The model under review builds one solid part; all positions refer to its coordinate system, in mm. Face numbers are marked on the shaded views. A direction names the side the tool comes from. Round coordinates to 2 decimals unless told otherwise and drop trailing zeros. Order: outer loops, then holes, each group sorted by start corner. A loop starts at its lowest first (then second) coordinate and runs counter-clockwise, first axis right, second up. Notation, with made-up numbers: M -6,40 L 43,40 A10 cw 43,56 Z; hole C 61.25,-23.75 d1. An arc over 180 degrees is marked long. Use a Markdown table: item, result. Add a question column.
1. For the marked faces 1, 2, 3, 4 and 5, list the 3-axis set-ups (+Z, -Z, +X, -X, +Y, -Y) from which the entire face can be reached by the end or side of a thin tool; tool diameter is ignored.
2. Consider section A-A on y = -43. State the section outline as (x, z) points.
3. The part is to be moulded in two halves that separate along Y. For the marked faces 6, 7, 8 and 9, say which applies: +Y half, -Y half, draft (parallel to the pull), parting line (faces both ways), or undercut.
4. Consider section C-C on x = 45. State the section outline as (y, z) points, then the cut area to 3 significant figures.
5. Consider section D-D on z = 22.5. State the section outline as (x, y) points.
6. Consider section B-B on z = 5.5. State the section outline as (x, y) points.
7. Insertion check: P1, Ø9, axis at x = -18, y = -40, coming from the +Z side; P2, Ø10, axis at x = 38.5, z = 22.5, coming from the -Y side; P3, Ø16.5, axis at x = 10.5, y = -27, coming from the +Z side; P4, Ø8, axis at x = 1, z = 15, coming from the +Y side. Each pin has a flat end and moves straight along its axis. Give the tip position at first contact, or say it passes through.
8. To check wall thickness, follow probe 1 along Y at (x, z) = (25.5, 0.5); probe 2 along Y at (x, z) = (0, 37.5); probe 3 along Z at (x, y) = (-11.5, -33). State the ranges of each line that lie inside material, in increasing order.
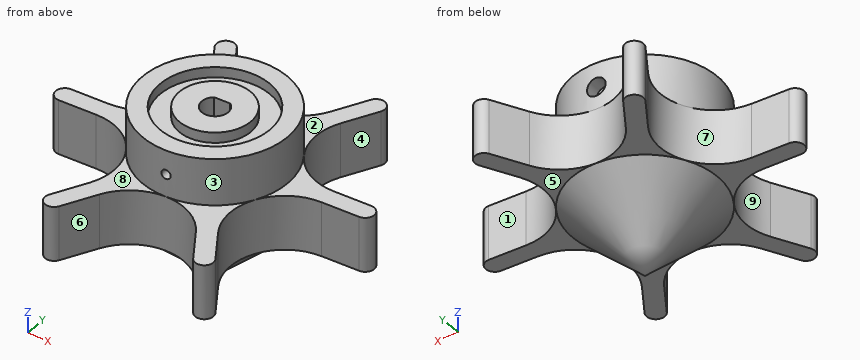
from build123d import *

# Parameters (mm, degrees)
SKETCH1_R               = 3.5
BOSS_EXTRUDE1_DEPTH     = 21
SKETCH4_R               = 28
BOSS_EXTRUDE2_DEPTH     = 18
SKETCH6_R               = 21.2
SKETCH6_R_2             = 13.8
CUT_EXTRUDE1_DEPTH      = 4
CUT_EXTRUDE2_DEPTH      = 20
CUT_EXTRUDE3_DEPTH      = 93.206949894
CUT_EXTRUDE3_DEPTH_BACK = 93.206949894
SKETCH7_R               = 1.75
SKETCH8_R               = 3.5
CUT_EXTRUDE4_DEPTH      = 5.5


with BuildPart() as part:
    # Sketch1 → Boss-Extrude1 (new body)
    with BuildSketch(Plane.XY):
        with BuildLine():
            ThreePointArc((-27.16441994, 47.550254291), (-29.67571676, 44.192804958), (-33.605829095, 45.653385243))
            Line((-33.605829095, 45.653385243), (-25.93972411, 33.765821671))
            ThreePointArc((-25.93972411, 33.765821671), (-24.90753088, 12.791204222), (-42.555985811, 1.409989939))
            Line((-42.555985811, 1.409989939), (-56.683970347, 0.71473006))
            ThreePointArc((-56.683970347, 0.71473006), (-54.098653318, -0.246072778), (-53.011938142, -2.781039515))
            ThreePointArc((-53.011938142, -2.781039515), (-53.976971405, -5.194324339), (-56.339905937, -6.27680909))
            Line((-56.339905937, -6.27680909), (-42.211921401, -5.581549211))
            ThreePointArc((-42.211921401, -5.581549211), (-23.531273241, -15.174952377), (-22.499080012, -36.149569826))
            Line((-22.499080012, -36.149569826), (-28.960959562, -48.732393278))
            ThreePointArc((-28.960959562, -48.732393278), (-25.025035607, -46.929305801), (-22.347518202, -50.331293805))
            ThreePointArc((-22.347518202, -50.331293805), (-22.445530198, -51.153776401), (-22.734076842, -51.930194333))
            Line((-22.734076842, -51.930194333), (-16.272197292, -39.347370882))
            ThreePointArc((-16.272197292, -39.347370882), (1.376257639, -27.966156599), (20.0569058, -37.559559765))
            Line((20.0569058, -37.559559765), (27.723010785, -49.447123338))
            ThreePointArc((27.723010785, -49.447123338), (28.767550893, -44.608845135), (33.605829095, -45.653385243))
            Line((33.605829095, -45.653385243), (25.93972411, -33.765821671))
            ThreePointArc((25.93972411, -33.765821671), (24.90753088, -12.791204222), (42.555985811, -1.409989939))
            Line((42.555985811, -1.409989939), (56.683970347, -0.71473006))
            ThreePointArc((56.683970347, -0.71473006), (53.016168567, 2.60900731), (56.339905937, 6.27680909))
            Line((56.339905937, 6.27680909), (42.211921401, 5.581549211))
            ThreePointArc((42.211921401, 5.581549211), (23.531273241, 15.174952377), (22.499080012, 36.149569826))
            Line((22.499080012, 36.149569826), (28.960959562, 48.732393278))
            ThreePointArc((28.960959562, 48.732393278), (24.248617674, 47.217852445), (22.734076842, 51.930194333))
            Line((22.734076842, 51.930194333), (16.272197292, 39.347370882))
            ThreePointArc((16.272197292, 39.347370882), (-1.376257639, 27.966156599), (-20.0569058, 37.559559765))
            Line((-20.0569058, 37.559559765), (-27.723010785, 49.447123338))
            ThreePointArc((-27.723010785, 49.447123338), (-27.306970607, 48.538957471), (-27.16441994, 47.550254291))
        make_face()
        with Locations((-56.511938142, -2.781039515)):
            Circle(SKETCH1_R)
        with Locations((-30.66441994, 47.550254291)):
            Circle(SKETCH1_R)
        with Locations((25.847518202, 50.331293805)):
            Circle(SKETCH1_R)
        with Locations((56.511938142, 2.781039515)):
            Circle(SKETCH1_R)
        with Locations((30.66441994, -47.550254291)):
            Circle(SKETCH1_R)
        with Locations((-25.847518202, -50.331293805)):
            Circle(SKETCH1_R)
    extrude(amount=BOSS_EXTRUDE1_DEPTH)

    # Sketch3 → Revolve1 (revolve)
    with BuildSketch(Plane(origin=(0, 0, 0), x_dir=(-0.9987913071010414, -0.04915205854685543, 0), z_dir=(0.04915205854685543, -0.9987913071010414, 0)), mode=Mode.PRIVATE) as revolve1_sk:
        Polygon((0, 0), (-28, 0), (0, 26.813467396), align=None)
    revolve(revolve1_sk.sketch.rotate(Axis((0, 0, -26.813467396), (0, 0, 1)), 357.182659299), axis=Axis((0, 0, -26.813467396), (0, 0, 1)))

    # Sketch4 → Boss-Extrude2 (add)
    with BuildSketch(Plane.XY.offset(21)):
        with Locations(Location((0, 0, 0), (0, 0, 152.817340701))):
            Circle(SKETCH4_R)
    extrude(amount=BOSS_EXTRUDE2_DEPTH)

    # Sketch6 → Cut-Extrude1 (cut)
    with BuildSketch(Plane.XY.offset(39)):
        Circle(SKETCH6_R)
        Circle(SKETCH6_R_2, mode=Mode.SUBTRACT)
    extrude(amount=-CUT_EXTRUDE1_DEPTH, mode=Mode.SUBTRACT)

    # Sketch5 → Cut-Extrude2 (cut)
    with BuildSketch(Plane.XY.offset(39)):
        with BuildLine():
            Line((2.82796059, 4.244129934), (-3.231007471, 3.945958784))
            ThreePointArc((-3.231007471, 3.945958784), (-2.183101223, -4.609128882), (5.1, 0))
            ThreePointArc((5.1, 0), (4.496253941, 2.407010697), (2.82796059, 4.244129934))
        make_face()
    extrude(amount=-CUT_EXTRUDE2_DEPTH, mode=Mode.SUBTRACT)

    # Sketch7 → Cut-Extrude3 (cut, two sides: drawn at the far end of the back side and taken through both)
    with BuildSketch(Plane(origin=(-0.20152344, 4.095044359, 0), x_dir=(0.9987913071010414, 0.049152058546853936, 0), z_dir=(0.049152058546853936, -0.9987913071010414, 0)).offset(-CUT_EXTRUDE3_DEPTH_BACK)):
        with Locations((0, 29.7)):
            Circle(SKETCH7_R)
    extrude(amount=CUT_EXTRUDE3_DEPTH + CUT_EXTRUDE3_DEPTH_BACK, mode=Mode.SUBTRACT)

    # Sketch8 → Cut-Extrude4 (cut)
    with BuildSketch(Plane(origin=(-1.376257639, 27.966156599, 0), x_dir=(0.9987913071010414, 0.049152058546855434, 0), z_dir=(-0.049152058546855434, 0.9987913071010414, 0))):
        with Locations(Location((0, -29.7, 0), (0, 0, 180))):
            Circle(SKETCH8_R)
    extrude(amount=-CUT_EXTRUDE4_DEPTH, mode=Mode.SUBTRACT)


solid = part.part
Answer block:
| question | item | result |
|---|---|---|
| 1 | face 1 | +Z, -Z, +Y |
| 1 | face 2 | +Z, +X, +Y |
| 1 | face 3 | +Z |
| 1 | face 4 | +Z, -Z, +X |
| 1 | face 5 | -Z, +X, +Y |
| 2 | outline | M -26.02,0 L -18.15,0 L -18.15,21 L -26.02,21 Z; M 23.57,0 L 31.89,0 L 31.89,21 L 23.57,21 Z |
| 3 | face 6 | -Y half |
| 3 | face 7 | undercut |
| 3 | face 8 | draft |
| 3 | face 9 | undercut |
| 4 | outline | M -1.29,0 L 5.72,0 L 5.72,21 L -1.29,21 Z |
| 4 | area | 147 mm^2 |
| 5 | outline | C 0,0 d56; hole M -3.23,3.95 A5.1 ccw long 2.83,4.24 Z |
| 6 | outline | M -56.68,0.71 A3.5 ccw -56.34,-6.28 L -42.21,-5.58 A21 cw -22.5,-36.15 L -28.96,-48.73 A3.5 ccw -22.73,-51.93 L -16.27,-39.35 A21 cw 20.06,-37.56 L 27.72,-49.45 A3.5 ccw 33.61,-45.65 L 25.94,-33.77 A21 cw 42.56,-1.41 L 56.68,-0.71 A3.5 ccw 56.34,6.28 L 42.21,5.58 A21 cw 22.5,36.15 L 28.96,48.73 A3.5 ccw 22.73,51.93 L 16.27,39.35 A21 cw -20.06,37.56 L -27.72,49.45 A3.5 ccw -33.61,45.65 L -25.94,33.77 A21 cw -42.56,1.41 Z |
| 7 | P1 | z = 21 |
| 7 | P2 | y = -49.24 |
| 7 | P3 | z = 39 |
| 7 | P4 | y = 29.29 |
| 8 | probe 1 | -46 to -33.05, -11.72 to 12.59, 41.99 to 53.81 |
| 8 | probe 2 | -28 to -21.2, -13.8 to -5.1, 4.1 to 13.8, 21.2 to 28 |
| 8 | probe 3 | 0 to 21 |
